Source: CAD feature listing. Evaluate the final solid. Frame: model axes, mm. A direction names the side the tool comes from. Give positions to 0.01 mm unless a question says otherwise; leave off trailing zeros. Order: outer loops, then holes, each group sorted by start corner. A loop starts at its lowest first (then second) coordinate and runs counter-clockwise, first axis right, second up. Notation, with made-up numbers: (6, -30.75) - (55, -30.75) arc R12 cw to (55, -9.75) - close; hole circle Ø10 at (-18, 45.25). An arc over 180 degrees is marked (long way). One line per item, written item: value. Start each with the question number.
from build123d import *

# Parameters (mm, degrees)
BOSS_EXTRUDE1_DEPTH    = 228.6
CONVERT_SOLID1_START   = -228.6
CONVERT_SOLID1_DEPTH   = 228.6
CONVERT_SOLID1_2_DEPTH = 228.6
SKETCH2_W              = 67.692558519
SKETCH2_H              = 152.4
SKETCH2_W_2            = 75.962864449
CUT_EXTRUDE1_DEPTH     = 244.449426781
SKETCH3_R              = 1.89865
CUT_EXTRUDE2_DEPTH     = 283.088699526
SKETCH4_R              = 2.2225
SKETCH4_R_2            = 1.89865
CUT_EXTRUDE3_DEPTH     = 244.449426781
SKETCH5_R              = 1.89865
CUT_EXTRUDE4_DEPTH     = 244.449426781
CUT_EXTRUDE5_DEPTH     = 244.379852289
SKETCH7_R              = 1.1
SKETCH7_R_2            = 1.05
CUT_EXTRUDE6_DEPTH     = 244.449426781
SKETCH8_R              = 1.37499852
CUT_EXTRUDE7_DEPTH     = 244.449426781
CUT_EXTRUDE8_DEPTH     = 244.449426781
SKETCH10_R             = 3.3
CUT_EXTRUDE9_DEPTH     = 244.449426781
FILLET1_R              = 5.08


# Read off the part's stored shape, not the designer's step: Convert-Solid1
with BuildPart() as part:
    # Sketch1 → Boss-Extrude1 (new body)
    with BuildSketch(Plane.XY):
        Polygon((82.55, 7.62), (82.55, -6.35), (81.28, -6.35), (81.28, 6.35), (-81.28, 6.35), (-81.28, -6.35), (-82.55, -6.35), (-82.55, 7.62), align=None)
    extrude(amount=-BOSS_EXTRUDE1_DEPTH)

    # Convert-Solid1 outline → Convert-Solid1 (cut)
    with BuildSketch(Plane.XY.offset(CONVERT_SOLID1_START)):
        with BuildLine():
            Line((82.55, 7.62), (80.01, 7.62))
            ThreePointArc((80.01, 7.62), (81.806051224, 6.876051224), (82.55, 5.08))
            Line((82.55, 5.08), (82.55, 7.62))
        make_face()
        with BuildLine():
            ThreePointArc((-82.55, 5.08), (-81.806051224, 6.876051224), (-80.01, 7.62))
            Line((-80.01, 7.62), (-82.55, 7.62))
            Line((-82.55, 7.62), (-82.55, 5.08))
        make_face()
    extrude(amount=CONVERT_SOLID1_DEPTH, mode=Mode.SUBTRACT)

    # Convert-Solid1 2 outline → Convert-Solid1 2 (add)
    with BuildSketch(Plane.XY.offset(CONVERT_SOLID1_START)):
        with BuildLine():
            Line((81.28, 6.35), (80.01, 6.35))
            ThreePointArc((80.01, 6.35), (80.908025612, 5.978025612), (81.28, 5.08))
            Line((81.28, 5.08), (81.28, 6.35))
        make_face()
        with BuildLine():
            ThreePointArc((-81.28, 5.08), (-80.908025612, 5.978025612), (-80.01, 6.35))
            Line((-80.01, 6.35), (-81.28, 6.35))
            Line((-81.28, 6.35), (-81.28, 5.08))
        make_face()
    extrude(amount=CONVERT_SOLID1_2_DEPTH)

    # Sketch2 → Cut-Extrude1 (cut, through all)
    with BuildSketch(Plane(origin=(0, 7.62, 0), x_dir=(1, 0, 0), z_dir=(0, 1, 0))):
        with Locations((-110.04627926, 101.6)):
            Rectangle(SKETCH2_W, SKETCH2_H)
        with Locations((114.181432225, 101.6)):
            Rectangle(SKETCH2_W_2, SKETCH2_H)
    extrude(amount=-CUT_EXTRUDE1_DEPTH, mode=Mode.SUBTRACT)

    # Sketch3 → Cut-Extrude2 (cut, through all)
    with BuildSketch(Plane.ZY.offset(82.55)):
        with Locations((-12.7, 0)):
            Circle(SKETCH3_R)
        with Locations((-190.498941664, 0)):
            Circle(SKETCH3_R)
    extrude(amount=-CUT_EXTRUDE2_DEPTH, mode=Mode.SUBTRACT)

    # Sketch4 → Cut-Extrude3 (cut, through all)
    with BuildSketch(Plane(origin=(0, 7.62, 0), x_dir=(1, 0, 0), z_dir=(0, 1, 0))):
        with Locations(Location((-66.230388698, 104.935772071, 0), (0, 0, 270))):
            Circle(SKETCH4_R)
        with Locations(Location((-66.230388698, 136.058157483, 0), (0, 0, 270))):
            Circle(SKETCH4_R)
        with Locations(Location((66.230388698, 104.943157483, 0), (0, 0, 270))):
            Circle(SKETCH4_R)
        with Locations(Location((66.230388698, 136.065542896, 0), (0, 0, 270))):
            Circle(SKETCH4_R)
        with Locations(Location((-64.77, 175.26, 0), (0, 0, 270))):
            Circle(SKETCH4_R_2)
        with Locations(Location((-29.765265396, 175.26, 0), (0, 0, 270))):
            Circle(SKETCH4_R_2)
        with Locations(Location((-64.77, 220.98, 0), (0, 0, 270))):
            Circle(SKETCH4_R_2)
        with Locations(Location((-29.765265396, 220.98, 0), (0, 0, 270))):
            Circle(SKETCH4_R_2)
    extrude(amount=-CUT_EXTRUDE3_DEPTH, mode=Mode.SUBTRACT)

    # Sketch5 → Cut-Extrude4 (cut, through all)
    with BuildSketch(Plane(origin=(0, 7.62, 0), x_dir=(1, 0, 0), z_dir=(0, 1, 0))):
        with Locations(Location((74.08, 215.385, 0), (0, 0, 270))):
            Circle(SKETCH5_R)
        with Locations(Location((74.08, 201.669, 0), (0, 0, 270))):
            Circle(SKETCH5_R)
    extrude(amount=-CUT_EXTRUDE4_DEPTH, mode=Mode.SUBTRACT)

    # Sketch6 → Cut-Extrude5 (cut, through all)
    with BuildSketch(Plane.XZ.offset(-6.35)):
        Polygon((7.397693639, -228.6), (7.397693639, -216.1), (30.897693639, -216.1), (30.897693639, -228.6), (32.459774255, -235.098021795), (8.736104366, -236.048499643), (7.834861371, -236.048499643), align=None)
    extrude(amount=-CUT_EXTRUDE5_DEPTH, mode=Mode.SUBTRACT)

    # Sketch7 → Cut-Extrude6 (cut, through all)
    with BuildSketch(Plane(origin=(0, 7.62, 0), x_dir=(1, 0, 0), z_dir=(0, 1, 0))):
        with Locations(Location((32.725, 222.7, 0), (0, 0, 270))):
            Circle(SKETCH7_R)
        with Locations(Location((5.025, 222.7, 0), (0, 0, 270))):
            Circle(SKETCH7_R_2)
    extrude(amount=-CUT_EXTRUDE6_DEPTH, mode=Mode.SUBTRACT)

    # Sketch8 → Cut-Extrude7 (cut, through all)
    with BuildSketch(Plane(origin=(0, 7.62, 0), x_dir=(1, 0, 0), z_dir=(0, 1, 0))):
        with Locations(Location((46.560590793, 146.00004873, 0), (0, 0, 270))):
            Circle(SKETCH8_R)
        with Locations(Location((-7.939606525, 144.005425812, 0), (0, 0, 270))):
            Circle(SKETCH8_R)
        with Locations(Location((-45.939409177, 146.009176787, 0), (0, 0, 270))):
            Circle(SKETCH8_R)
        with Locations(Location((-45.947797121, 61.009177021, 0), (0, 0, 270))):
            Circle(SKETCH8_R)
        with Locations(Location((-2.447795433, 61.004884367, 0), (0, 0, 270))):
            Circle(SKETCH8_R)
        with Locations(Location((46.552202848, 61.000048964, 0), (0, 0, 270))):
            Circle(SKETCH8_R)
        with Locations(Location((46.54647931, 3.000048406, 0), (0, 0, 270))):
            Circle(SKETCH8_R)
        with Locations(Location((-2.453518972, 3.00488381, 0), (0, 0, 270))):
            Circle(SKETCH8_R)
        with Locations(Location((-45.95352066, 3.009176464, 0), (0, 0, 270))):
            Circle(SKETCH8_R)
    extrude(amount=-CUT_EXTRUDE7_DEPTH, mode=Mode.SUBTRACT)

    # Sketch9 → Cut-Extrude8 (cut, through all)
    with BuildSketch(Plane(origin=(0, 7.62, 0), x_dir=(1, 0, 0), z_dir=(0, 1, 0))):
        with BuildLine():
            Line((-62.23, 92.71), (-57.15, 92.71))
            ThreePointArc((-57.15, 92.71), (-53.557897552, 91.222102448), (-52.07, 87.63))
            Line((-52.07, 87.63), (-52.07, 40.64))
            ThreePointArc((-52.07, 40.64), (-53.557897552, 37.047897552), (-57.15, 35.56))
            Line((-57.15, 35.56), (-62.23, 35.56))
            ThreePointArc((-62.23, 35.56), (-65.822102448, 37.047897552), (-67.31, 40.64))
            Line((-67.31, 40.64), (-67.31, 87.63))
            ThreePointArc((-67.31, 87.63), (-65.822102448, 91.222102448), (-62.23, 92.71))
        make_face()
    extrude(amount=-CUT_EXTRUDE8_DEPTH, mode=Mode.SUBTRACT)

    # Sketch10 → Cut-Extrude9 (cut, through all)
    with BuildSketch(Plane(origin=(0, 7.62, 0), x_dir=(1, 0, 0), z_dir=(0, 1, 0))):
        with Locations(Location((62.23, 12.7, 0), (0, 0, 270))):
            Circle(SKETCH10_R)
        with Locations(Location((62.23, 29.21, 0), (0, 0, 270))):
            Circle(SKETCH10_R)
        with Locations(Location((62.23, 45.72, 0), (0, 0, 270))):
            Circle(SKETCH10_R)
        with Locations(Location((62.23, 62.23, 0), (0, 0, 270))):
            Circle(SKETCH10_R)
        with Locations(Location((62.23, 78.74, 0), (0, 0, 270))):
            Circle(SKETCH10_R)
    extrude(amount=-CUT_EXTRUDE9_DEPTH, mode=Mode.SUBTRACT)

    # Fillet1
    fillet1_edges = [part.edges().sort_by_distance(p)[0] for p in [
        (81.915, -6.35, 0),
        (81.915, -6.35, -228.6),
        (-81.915, -6.35, -228.6),
        (-81.915, -6.35, 0),
        (-81.915, -6.35, -25.4),
        (-81.915, -6.35, -177.8),
        (81.915, -6.35, -25.4),
        (81.915, -6.35, -177.8),
    ]]
    fillet(fillet1_edges, radius=FILLET1_R)


solid = part.part
1. Section A-A on z = -29.21. Return the cut outline in (x, y), then the cut area to 3 significant figures.
2. Draft query along X for faces 4 (the cylindrical face through (60.97, 6.99, -42.67)), 5 (the flat face through (-82.55, -1, -203)), 6 (the flat face through (81.5, 4.5, -177.8)). Return one class per face: pulls with the +X half, pulls with the -X half, needs draft (parallel to the pull), parting line crosses it, or undercut.
3. Contact query for flat-ended pins moving along their axis: pin 1 Ø3 at (x, z) = (-2.45, -3) entering from +Y; pin 2 Ø10.5 at (x, z) = (62.23, -12.7) entering from -Y; pin 3 Ø1.4 at (x, y) = (14, 7) entering from -Z; pin 4 Ø1 at (y, z) = (6.5, -69.5) entering from -X. Output: stop coordinate, or through.
4. Ray query, L1, parallel to X at y = 4, z = -10; L2, parallel to X at y = 7.1, z = -78.74; L3, parallel to Y at x = 50.5, z = -26. Return the intervals inside material, ascending.
5. Set-up query: faces 1 (the cylindrical face through (81.924, -4.822, -179.249)), 2 (the flat face through (-82, 5, -177.8)), 3 (the flat face through (81.28, -1, -203)). Return all of +Z, -Z, +X, -X, +Y, -Y with unobstructed straight access to the full face (end or side cutting, diameter ignored); none if empty.
Data:
1. outline: (-76.2, 6.35) - (58.93, 6.35) - (58.93, 7.62) - (-76.2, 7.62) - close; (65.53, 6.35) - (76.2, 6.35) - (76.2, 7.62) - (65.53, 7.62) - close
1. area: 185 mm2
2. face 4: undercut
2. face 5: pulls with the -X half
2. face 6: needs draft
3. pin 1: stops at y = 7.62
3. pin 2: stops at y = 6.35
3. pin 3: stops at z = -216.1
3. pin 4: stops at x = -76.2
4. L1: x = -82.55 to -81.28, 81.28 to 82.55
4. L2: x = -76.2 to -67.31, -52.07 to 58.93, 65.53 to 76.2
4. L3: y = 6.35 to 7.62
5. face 1: +X, -X, -Y
5. face 2: -X, +Y, -Y
5. face 3: +Z, -Z, -Y
